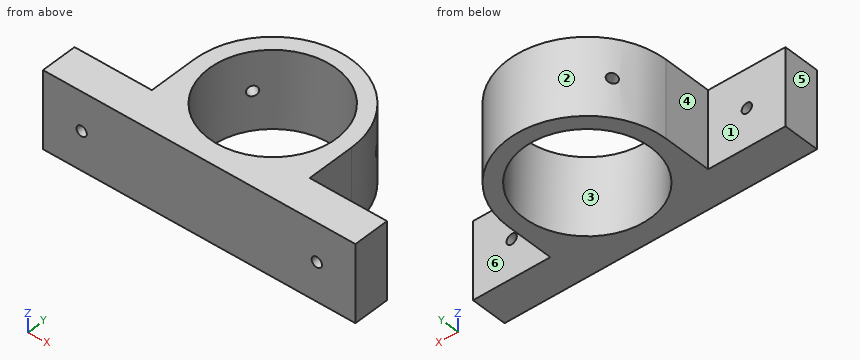
```python
from build123d import *

# Parameters (mm, degrees)
BOSS_EXTRUDE1_DEPTH = 15
BOSS_EXTRUDE2_START = -15
BOSS_EXTRUDE2_DEPTH = 15
SKETCH2_R           = 1
CUT_EXTRUDE1_DEPTH  = 25
SKETCH5_R           = 1
CUT_EXTRUDE2_DEPTH  = 4
SKETCH6_R           = 1
CUT_EXTRUDE3_DEPTH  = 4


with BuildPart() as part:
    # Sketch1 → Boss-Extrude1 (new body)
    with BuildSketch(Plane.XY):
        with BuildLine():
            Line((-12.31, 0), (-12.31, -12.31))
            Line((-12.31, -12.31), (-30.31, -12.31))
            Line((-30.31, -12.31), (-30.31, -9.31))
            Line((-30.31, -9.31), (-15.31, -9.31))
            Line((-15.31, -9.31), (-15.31, 0))
            ThreePointArc((-15.31, 0), (0, 15.31), (15.31, 0))
            Line((15.31, 0), (15.31, -9.31))
            Line((15.31, -9.31), (30.31, -9.31))
            Line((30.31, -9.31), (30.31, -12.31))
            Line((30.31, -12.31), (12.31, -12.31))
            Line((12.31, -12.31), (12.31, 0))
            ThreePointArc((12.31, 0), (0, 12.31), (-12.31, 0))
        make_face()
    extrude(amount=BOSS_EXTRUDE1_DEPTH)

    # Sketch3 → Boss-Extrude2 (add)
    with BuildSketch(Plane.XY.offset(15).offset(BOSS_EXTRUDE2_START)):
        with BuildLine():
            Line((-30.31, -12.31), (-12.31, -12.31))
            Line((-12.31, -12.31), (-12.31, 0))
            ThreePointArc((-12.31, 0), (0, -12.31), (12.31, 0))
            Line((12.31, 0), (12.31, -12.31))
            Line((12.31, -12.31), (30.31, -12.31))
            Line((30.31, -12.31), (30.31, -16.31))
            Line((30.31, -16.31), (-30.31, -16.31))
            Line((-30.31, -16.31), (-30.31, -12.31))
        make_face()
    extrude(amount=BOSS_EXTRUDE2_DEPTH)

    # Sketch2 → Cut-Extrude1 (cut)
    with BuildSketch(Plane(origin=(0, -9.31, 0), x_dir=(1, 0, 0), z_dir=(0, 1, 0))):
        with Locations(Location((22.81, -7.5, 0), (0, 0, 270))):
            Circle(SKETCH2_R)
        with Locations(Location((-22.81, -7.5, 0), (0, 0, 270))):
            Circle(SKETCH2_R)
    extrude(amount=-CUT_EXTRUDE1_DEPTH, mode=Mode.SUBTRACT)

    # Sketch5 → Cut-Extrude2 (cut)
    with BuildSketch(Plane(origin=(12.541217798, 8.781455241, 0), x_dir=(0, 0, -1), z_dir=(0.819152044288993, 0.5735764363510446, 0))):
        with Locations(Location((-7.5, 0, 0), (0, 0, 90))):
            Circle(SKETCH5_R)
    extrude(amount=-CUT_EXTRUDE2_DEPTH, mode=Mode.SUBTRACT)

    # Sketch6 → Cut-Extrude3 (cut)
    with BuildSketch(Plane(origin=(-12.541217798, 8.781455241, 0), x_dir=(0, 0, 1), z_dir=(-0.8191520442889931, 0.5735764363510442, 0))):
        with Locations(Location((7.5, 0, 0), (0, 0, 270))):
            Circle(SKETCH6_R)
    extrude(amount=-CUT_EXTRUDE3_DEPTH, mode=Mode.SUBTRACT)


solid = part.part
```
Geometry check sheet. Reference: the model listing, model coordinates, mm. Face numbers are marked on the shaded views. A direction names the side the tool comes from. Coordinates: 2 decimals unless noted, no trailing zeros. Loops run counter-clockwise (first coordinate to the right, second up) from the corner with the lowest first, then second, coordinate; pieces in that order, holes last. Notation, with made-up numbers: (-5.75, -10.75) - (10.25, -10.75) arc R13 ccw to (10.25, 8.25) - close; hole circle Ø11 at (-1.5, 89.25). An arc over 180 degrees is marked (long way). One line per item, written item: value. Start each with the question number.
(1) Cross-section at A-A on y = -11.5. Enter the section's corners in (x, z), plus the area to 3 significant figures.
(2) Material ranges on line 1 (X direction, y = -13.5, z = 7.5); line 2 (Y direction, x = -5.5, z = 11.5); line 3 (X direction, y = -11, z = 7.5), recorded low to high. Write a range as [from, to].
(3) Cross-section at D-D on y = -8. Enter the section's corners in (x, z), plus the area to 3 significant figures.
(4) Depth check by flat-ended pin: P1, Ø5, axis at y = 8, z = 4.5, coming from the -X side; P2, Ø4.5, axis at y = -5, z = 4, coming from the -X side; P3, Ø4.5, axis at y = -3.5, z = 6, coming from the +X side. Enter the tip coordinate at first touch or a pass-through.
(5) Cross-section at B-B on x = -22.81. Enter the section's corners in (y, z).
(6) Cross-section at C-C on z = 7.5. Enter the section's corners in (x, y), plus the area to 3 significant figures.
(7) Mould release check, pull along X, two halves, no side actions. Record for the marked faces 1, 2, 3 and 4: released by +X, released by -X, zero draft, split by the parting line, or undercut.
(8) Tool access check on the marked faces 5 and 6. Record the directions out of +Z, -Z, +X, -X, +Y, -Y that give a thin tool (end or side, any length) a straight path to the whole face; none if there is none.
Results below:
1. outline: (-30.31, 0) - (-4.39, 0) - (-4.39, 15) - (-30.31, 15) - close; (4.39, 0) - (30.31, 0) - (30.31, 15) - (4.39, 15) - close; hole circle Ø2 at (-22.81, 7.5); hole circle Ø2 at (22.81, 7.5)
1. area: 771 mm2
2. line 1: x = [-30.31, -23.81], [-21.81, 21.81], [23.81, 30.31]
2. line 2: y = [-16.31, -11.01], [11.01, 14.29]
2. line 3: x = [-30.31, -23.81], [-21.81, -5.53], [5.53, 21.81], [23.81, 30.31]
3. outline: (-15.31, 0) - (-9.36, 0) - (-9.36, 15) - (-15.31, 15) - close; (9.36, 0) - (15.31, 0) - (15.31, 15) - (9.36, 15) - close
3. area: 179 mm2
4. P1: stops at x = -14.29
4. P2: stops at x = -15.31
4. P3: stops at x = 15.31
5. outline: (-16.31, 0) - (-9.31, 0) - (-9.31, 6.5) - (-16.31, 6.5) - close; (-16.31, 8.5) - (-9.31, 8.5) - (-9.31, 15) - (-16.31, 15) - close
6. outline: (-30.31, -16.31) - (-23.81, -16.31) - (-23.81, -9.31) - (-30.31, -9.31) - close; (-21.81, -16.31) - (21.81, -16.31) - (21.81, -9.31) - (15.31, -9.31) - (15.31, 0) arc R15.31 ccw to (13.09, 7.94) - (10.62, 6.22) arc R12.31 cw (long way) to (-10.62, 6.22) - (-13.09, 7.94) arc R15.31 ccw to (-15.31, 0) - (-15.31, -9.31) - (-21.81, -9.31) - close; (-11.94, 9.58) - (-9.48, 7.86) arc R12.31 cw to (9.48, 7.86) - (11.94, 9.58) arc R15.31 ccw to start; (23.81, -16.31) - (30.31, -16.31) - (30.31, -9.31) - (23.81, -9.31) - close
6. area: 562 mm2
7. face 1: zero draft
7. face 2: split by the parting line
7. face 3: undercut
7. face 4: released by -X
8. face 5: +Z, -Z, -X, +Y, -Y
8. face 6: +Z, -Z, +X, +Y
